from build123d import *

# Parameters (mm, degrees)
IZIM1_W                     = 300
IZIM1_H                     = 100
Y_KSEKLIK_EKSTR_ZYON1_DEPTH = 200
BO_ALTMA1_T                 = -4
KES_EKSTR_ZYON1_REACH       = 376.166
IZIM2_R                     = 4
KES_EKSTR_ZYON2_REACH       = 376.166
IZIM3_R                     = 2
IZIM3_W                     = 40
IZIM3_H                     = 20


with BuildPart() as part:
    # Çizim1 → Yükseklik-Ekstrüzyon1 (new body)
    with BuildSketch(Plane.XY):
        with Locations((-150, 50)):
            Rectangle(IZIM1_W, IZIM1_H)
    extrude(amount=Y_KSEKLIK_EKSTR_ZYON1_DEPTH)

    # İç Boşaltma1
    bo_altma1_openings = [part.faces().sort_by_distance(p)[0] for p in [
        (-300, 50, 100),
        (0, 50, 100),
    ]]
    offset(amount=BO_ALTMA1_T, openings=bo_altma1_openings, kind=Kind.INTERSECTION)

    # Çizim2 → Kes-Ekstrüzyon1 (cut, up to next)
    with BuildSketch(Plane.XZ, mode=Mode.PRIVATE) as kes_ekstr_zyon1_sk1:
        with Locations((-271.25, 146.25)):
            Circle(IZIM2_R)
    kes_ekstr_zyon1_tool1 = extrude(kes_ekstr_zyon1_sk1.sketch, amount=-KES_EKSTR_ZYON1_REACH, mode=Mode.PRIVATE) & part.part
    # Çizim2 → Kes-Ekstrüzyon1 (cut, up to next)
    with BuildSketch(Plane.XZ, mode=Mode.PRIVATE) as kes_ekstr_zyon1_sk2:
        with Locations((-178.75, 146.25)):
            Circle(IZIM2_R)
    kes_ekstr_zyon1_tool2 = extrude(kes_ekstr_zyon1_sk2.sketch, amount=-KES_EKSTR_ZYON1_REACH, mode=Mode.PRIVATE) & part.part
    # Çizim2 → Kes-Ekstrüzyon1 (cut, up to next)
    with BuildSketch(Plane.XZ, mode=Mode.PRIVATE) as kes_ekstr_zyon1_sk3:
        with Locations(Location((-28.75, 146.25, 0), (0, 0, 180))):
            Circle(IZIM2_R)
    kes_ekstr_zyon1_tool3 = extrude(kes_ekstr_zyon1_sk3.sketch, amount=-KES_EKSTR_ZYON1_REACH, mode=Mode.PRIVATE) & part.part
    # Çizim2 → Kes-Ekstrüzyon1 (cut, up to next)
    with BuildSketch(Plane.XZ, mode=Mode.PRIVATE) as kes_ekstr_zyon1_sk4:
        with Locations(Location((-121.25, 146.25, 0), (0, 0, 180))):
            Circle(IZIM2_R)
    kes_ekstr_zyon1_tool4 = extrude(kes_ekstr_zyon1_sk4.sketch, amount=-KES_EKSTR_ZYON1_REACH, mode=Mode.PRIVATE) & part.part
    # Çizim2 → Kes-Ekstrüzyon1 (cut, up to next)
    with BuildSketch(Plane.XZ, mode=Mode.PRIVATE) as kes_ekstr_zyon1_sk5:
        with Locations((-271.25, 53.75)):
            Circle(IZIM2_R)
    kes_ekstr_zyon1_tool5 = extrude(kes_ekstr_zyon1_sk5.sketch, amount=-KES_EKSTR_ZYON1_REACH, mode=Mode.PRIVATE) & part.part
    # Çizim2 → Kes-Ekstrüzyon1 (cut, up to next)
    with BuildSketch(Plane.XZ, mode=Mode.PRIVATE) as kes_ekstr_zyon1_sk6:
        with Locations((-178.75, 53.75)):
            Circle(IZIM2_R)
    kes_ekstr_zyon1_tool6 = extrude(kes_ekstr_zyon1_sk6.sketch, amount=-KES_EKSTR_ZYON1_REACH, mode=Mode.PRIVATE) & part.part
    # Çizim2 → Kes-Ekstrüzyon1 (cut, up to next)
    with BuildSketch(Plane.XZ, mode=Mode.PRIVATE) as kes_ekstr_zyon1_sk7:
        with Locations(Location((-121.25, 53.75, 0), (0, 0, 180))):
            Circle(IZIM2_R)
    kes_ekstr_zyon1_tool7 = extrude(kes_ekstr_zyon1_sk7.sketch, amount=-KES_EKSTR_ZYON1_REACH, mode=Mode.PRIVATE) & part.part
    # Çizim2 → Kes-Ekstrüzyon1 (cut, up to next)
    with BuildSketch(Plane.XZ, mode=Mode.PRIVATE) as kes_ekstr_zyon1_sk8:
        with Locations(Location((-28.75, 53.75, 0), (0, 0, 180))):
            Circle(IZIM2_R)
    kes_ekstr_zyon1_tool8 = extrude(kes_ekstr_zyon1_sk8.sketch, amount=-KES_EKSTR_ZYON1_REACH, mode=Mode.PRIVATE) & part.part
    add(kes_ekstr_zyon1_tool1.solids().sort_by_distance((-271.25, 0, 146.25))[0], mode=Mode.SUBTRACT)
    add(kes_ekstr_zyon1_tool2.solids().sort_by_distance((-178.75, 0, 146.25))[0], mode=Mode.SUBTRACT)
    add(kes_ekstr_zyon1_tool3.solids().sort_by_distance((-28.75, 0, 146.25))[0], mode=Mode.SUBTRACT)
    add(kes_ekstr_zyon1_tool4.solids().sort_by_distance((-121.25, 0, 146.25))[0], mode=Mode.SUBTRACT)
    add(kes_ekstr_zyon1_tool5.solids().sort_by_distance((-271.25, 0, 53.75))[0], mode=Mode.SUBTRACT)
    add(kes_ekstr_zyon1_tool6.solids().sort_by_distance((-178.75, 0, 53.75))[0], mode=Mode.SUBTRACT)
    add(kes_ekstr_zyon1_tool7.solids().sort_by_distance((-121.25, 0, 53.75))[0], mode=Mode.SUBTRACT)
    add(kes_ekstr_zyon1_tool8.solids().sort_by_distance((-28.75, 0, 53.75))[0], mode=Mode.SUBTRACT)

    # Çizim3 → Kes-Ekstrüzyon2 (cut, up to next)
    with BuildSketch(Plane(origin=(0, 100, 0), x_dir=(1, 0, 0), z_dir=(0, 1, 0)), mode=Mode.PRIVATE) as kes_ekstr_zyon2_sk1:
        with Locations(Location((-116.5, -95, 0), (0, 0, 180))):
            Circle(IZIM3_R)
    kes_ekstr_zyon2_tool1 = extrude(kes_ekstr_zyon2_sk1.sketch, amount=-KES_EKSTR_ZYON2_REACH, mode=Mode.PRIVATE) & part.part
    # Çizim3 → Kes-Ekstrüzyon2 (cut, up to next)
    with BuildSketch(Plane(origin=(0, 100, 0), x_dir=(1, 0, 0), z_dir=(0, 1, 0)), mode=Mode.PRIVATE) as kes_ekstr_zyon2_sk2:
        with Locations(Location((-116.5, -105, 0), (0, 0, 180))):
            Circle(IZIM3_R)
    kes_ekstr_zyon2_tool2 = extrude(kes_ekstr_zyon2_sk2.sketch, amount=-KES_EKSTR_ZYON2_REACH, mode=Mode.PRIVATE) & part.part
    # Çizim3 → Kes-Ekstrüzyon2 (cut, up to next)
    with BuildSketch(Plane(origin=(0, 100, 0), x_dir=(1, 0, 0), z_dir=(0, 1, 0)), mode=Mode.PRIVATE) as kes_ekstr_zyon2_sk3:
        with Locations(Location((-163.5, -105, 0), (0, 0, 180))):
            Circle(IZIM3_R)
    kes_ekstr_zyon2_tool3 = extrude(kes_ekstr_zyon2_sk3.sketch, amount=-KES_EKSTR_ZYON2_REACH, mode=Mode.PRIVATE) & part.part
    # Çizim3 → Kes-Ekstrüzyon2 (cut, up to next)
    with BuildSketch(Plane(origin=(0, 100, 0), x_dir=(1, 0, 0), z_dir=(0, 1, 0)), mode=Mode.PRIVATE) as kes_ekstr_zyon2_sk4:
        with Locations(Location((-163.5, -95, 0), (0, 0, 180))):
            Circle(IZIM3_R)
    kes_ekstr_zyon2_tool4 = extrude(kes_ekstr_zyon2_sk4.sketch, amount=-KES_EKSTR_ZYON2_REACH, mode=Mode.PRIVATE) & part.part
    # Çizim3 → Kes-Ekstrüzyon2 (cut, up to next)
    with BuildSketch(Plane(origin=(0, 100, 0), x_dir=(1, 0, 0), z_dir=(0, 1, 0)), mode=Mode.PRIVATE) as kes_ekstr_zyon2_sk5:
        with Locations((-140, -100)):
            Rectangle(IZIM3_W, IZIM3_H)
    kes_ekstr_zyon2_tool5 = extrude(kes_ekstr_zyon2_sk5.sketch, amount=-KES_EKSTR_ZYON2_REACH, mode=Mode.PRIVATE) & part.part
    add(kes_ekstr_zyon2_tool1.solids().sort_by_distance((-116.5, 100, 95))[0], mode=Mode.SUBTRACT)
    add(kes_ekstr_zyon2_tool2.solids().sort_by_distance((-116.5, 100, 105))[0], mode=Mode.SUBTRACT)
    add(kes_ekstr_zyon2_tool3.solids().sort_by_distance((-163.5, 100, 105))[0], mode=Mode.SUBTRACT)
    add(kes_ekstr_zyon2_tool4.solids().sort_by_distance((-163.5, 100, 95))[0], mode=Mode.SUBTRACT)
    add(kes_ekstr_zyon2_tool5.solids().sort_by_distance((-140, 100, 100))[0], mode=Mode.SUBTRACT)


solid = part.part
Work out the finished part from the listing and answer in its coordinate system (mm). A direction names the side the tool comes from. Round coordinates to 2 decimals unless told otherwise and drop trailing zeros. Write each loop counter-clockwise with the first axis right and the second up, starting at its lowest first coordinate (ties: lowest second). Pieces come first, ordered by that corner, then holes.
1) Straight lines are drawn through the part: line 1 (Z direction, x = -116.5, y = 98.35); line 2 (Z direction, x = -28.75, y = 3.25); line 3 (Z direction, x = -65, y = 80.5). For each, find the intervals that lie inside material, in ascending order.
2) A cutting plane is placed at A-A (x = -178.75). Give the vertices of the cut face in (y, z).
3) The mould has two halves that part along Y. Classify faces 1 (the flat face through (-152, 51, 4)), 2 (the flat face through (-152, 100, 76)), 3 (the cylindrical face through (-120.729, 1.972, 142.284)): pulls with the +Y half, pulls with the -Y half, needs draft (parallel to the pull), parting line crosses it, or undercut.
4) A cutting plane is placed at C-C (z = 146.25). Give the vertices of the cut face in (x, y), plus the area to 3 significant figures.
5) A cutting plane is placed at B-B (y = 39). Give the vertices of the cut face in (x, z), plus the area to 3 significant figures.
6) A cutting plane is placed at D-D (x = -99). Give the vertices of the cut face in (y, z).
7) A tool of negligible diameter and unlimited length cuts with its end or side. For faces 4 (the cylindrical face through (-176.6, 1.972, 149.623)), 5 (the flat face through (-152, 51, 196)), 6 (the flat face through (-300, 2, 70)), from which of +Z, -Z, +X, -X, +Y, -Y can it reach the whole face along a straight path? Write none if from no direction.
Completed:
1. line 1: z = 0 to 93, 97 to 103, 107 to 200
1. line 2: z = 0 to 49.75, 57.75 to 142.25, 150.25 to 200
1. line 3: z = 0 to 4, 196 to 200
2. outline: (0, 0) - (100, 0) - (100, 200) - (0, 200) - (0, 150.25) - (4, 150.25) - (4, 196) - (96, 196) - (96, 4) - (4, 4) - (4, 49.75) - (0, 49.75) - close; (0, 57.75) - (4, 57.75) - (4, 142.25) - (0, 142.25) - close
3. face 1: undercut
3. face 2: pulls with the +Y half
3. face 3: needs draft
4. outline: (-300, 0) - (-275.25, 0) - (-275.25, 4) - (-300, 4) - close; (-300, 96) - (0, 96) - (0, 100) - (-300, 100) - close; (-267.25, 0) - (-182.75, 0) - (-182.75, 4) - (-267.25, 4) - close; (-174.75, 0) - (-125.25, 0) - (-125.25, 4) - (-174.75, 4) - close; (-117.25, 0) - (-32.75, 0) - (-32.75, 4) - (-117.25, 4) - close; (-24.75, 0) - (0, 0) - (0, 4) - (-24.75, 4) - close
4. area: 2,270 mm2
5. outline: (-300, 0) - (0, 0) - (0, 4) - (-300, 4) - close; (-300, 196) - (0, 196) - (0, 200) - (-300, 200) - close
5. area: 2,400 mm2
6. outline: (0, 0) - (100, 0) - (100, 200) - (0, 200) - close; hole (4, 4) - (96, 4) - (96, 196) - (4, 196) - close
7. face 4: -Y
7. face 5: +X, -X
7. face 6: +Z, -Z, -X, +Y, -Y
